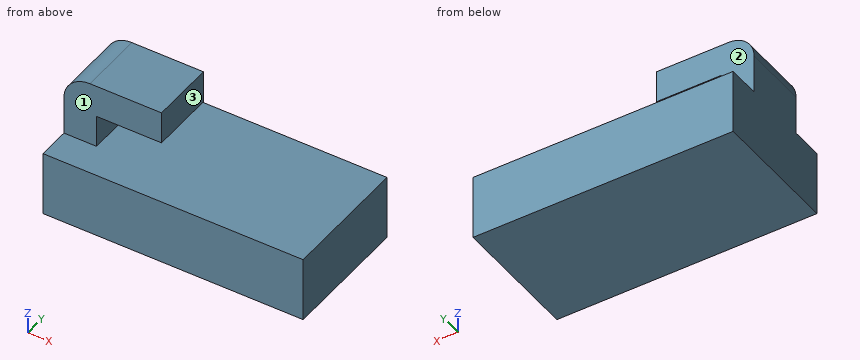
```python
from build123d import *

# Parameters (mm, degrees)
F0_W     = 50.8
F0_H     = 25.4
F1_DEPTH = 12.7
F2_W     = 19.05
F2_H     = 12.7
F3_DEPTH = 12.7
F4_W     = 12.7
F4_H     = 6.35
F5_DEPTH = 12.7
F6_R     = 5.08


with BuildPart() as f1:
    # F0 (on Top) → F1 (new body)
    with BuildSketch(Plane.XY):
        with Locations((-5.801945, -1.255406)):
            Rectangle(F0_W, F0_H)
    extrude(amount=F1_DEPTH)

    # F2 (on face) → F3 (join)
    with BuildSketch(Plane.XY.offset(12.7)):
        with Locations((-21.676945, -1.255406)):
            Rectangle(F2_W, F2_H)
    extrude(amount=F3_DEPTH)

    # F4 (on face) → F5 (cut, through all)
    with BuildSketch(Plane.XZ.offset(7.605406)):
        with Locations((-18.501945, 15.875)):
            Rectangle(F4_W, F4_H)
    extrude(amount=-F5_DEPTH, mode=Mode.SUBTRACT)

    # F6
    f6_edges = [f1.edges().sort_by_distance(p)[0] for p in [
        (-31.201945, -1.255406, 25.4),
    ]]
    fillet(f6_edges, radius=F6_R)


solid = f1.part
```
For this review, take the finished solid that the model builds, in its own axes (mm). Face numbers are marked on the shaded views. A direction names the side the tool comes from. Give positions to 0.01 mm unless a question says otherwise; leave off trailing zeros. Write each loop counter-clockwise with the first axis right and the second up, starting at its lowest first coordinate (ties: lowest second). Pieces come first, ordered by that corner, then holes. Notation, with made-up numbers: M -32.5,25 L 9.5,25 A34 ccw 9.5,57 Z; hole C 51,61 d6. An arc over 180 degrees is marked long. Answer as CSV lines item,"result".
1. For pin 1 (3 mm diameter, centred on y = 8.5, z = 15.5, fed in from -X); pin 2 (3 mm diameter, centred on x = 1, y = -3.5, fed in from +Z); pin 3 (1 mm diameter, centred on y = -2.5, z = 21, fed in from -X); pin 4 (7 mm diameter, centred on y = -3, z = 17, fed in from +X), all flat-tipped, find the tip position at first contact; note any pin that passes through.
Findings:
pin 1,"passes through"
pin 2,"stops at z = 12.7"
pin 3,"stops at x = -31.2"
pin 4,"stops at x = -12.15"
2. For the marked faces 1, 2 and 3, list the 3-axis set-ups (+Z, -Z, +X, -X, +Y, -Y) from which the entire face can be reached by the end or side of a thin tool; tool diameter is ignored.
Findings:
face 1,"+Z, +X, -X, -Y"
face 2,"+Z, +X, -X, +Y"
face 3,"+Z, +X, +Y, -Y"
3. Consider section D-D, the plane y = 5.75. Write out the cut boundary in (x, z), then the cut area to 3 significant figures.
Findings:
outline,"M -31.2,0 L 19.6,0 L 19.6,12.7 L -31.2,12.7 Z"
area,"645 mm2"
4. Consider section C-C, the plane x = -28. Write out the cut boundary in (y, z).
Findings:
outline,"M -13.96,0 L 11.44,0 L 11.44,12.7 L 5.09,12.7 L 5.09,25.04 L -7.61,25.04 L -7.61,12.7 L -13.96,12.7 Z"
5. Consider section A-A, the plane x = -13. Write out the cut boundary in (y, z), then the cut area to 3 significant figures.
Findings:
outline,"M -13.96,0 L 11.44,0 L 11.44,12.7 L -13.96,12.7 Z; M -7.61,19.05 L 5.09,19.05 L 5.09,25.4 L -7.61,25.4 Z"
area,"403 mm2"
6. Consider section B-B, the plane y = -6.75. Write out the cut boundary in (x, z), then the cut area to 3 significant figures.
Findings:
outline,"M -31.2,0 L 19.6,0 L 19.6,12.7 L -24.85,12.7 L -24.85,19.05 L -12.15,19.05 L -12.15,25.4 L -26.12,25.4 A5.08 ccw -31.2,20.32 Z"
area,"801 mm2"
7. Wall thickness on line 1 (Z direction, x = -12.5, y = 2.5); line 2 (Z direction, x = 10.5, y = -2.75); line 3 (X direction, y = -3.75, z = 20): over which ranges is each line inside the solid? List them lowest first.
Findings:
line 1,"z = 0 to 12.7, 19.05 to 25.4"
line 2,"z = 0 to 12.7"
line 3,"x = -31.2 to -12.15"
